The figure shows three views and two pictorial views of one solid part (mm, origin at its lowest corner). Answer the questions. A direction names the side the tool comes from. Give positions to 0.01 mm unless a question says otherwise; leave off trailing zeros. Order: outer loops, then holes, each group sorted by start corner. A loop starts at its lowest first (then second) coordinate and runs counter-clockwise, first axis right, second up. Notation, with made-up numbers: (8.5, 0.25) - (40.5, 0.25) arc R15 ccw to (40.5, 5.25) - close; hole circle Ø11 at (-1.75, 50). An arc over 180 degrees is marked (long way). Write item = value, one per line.
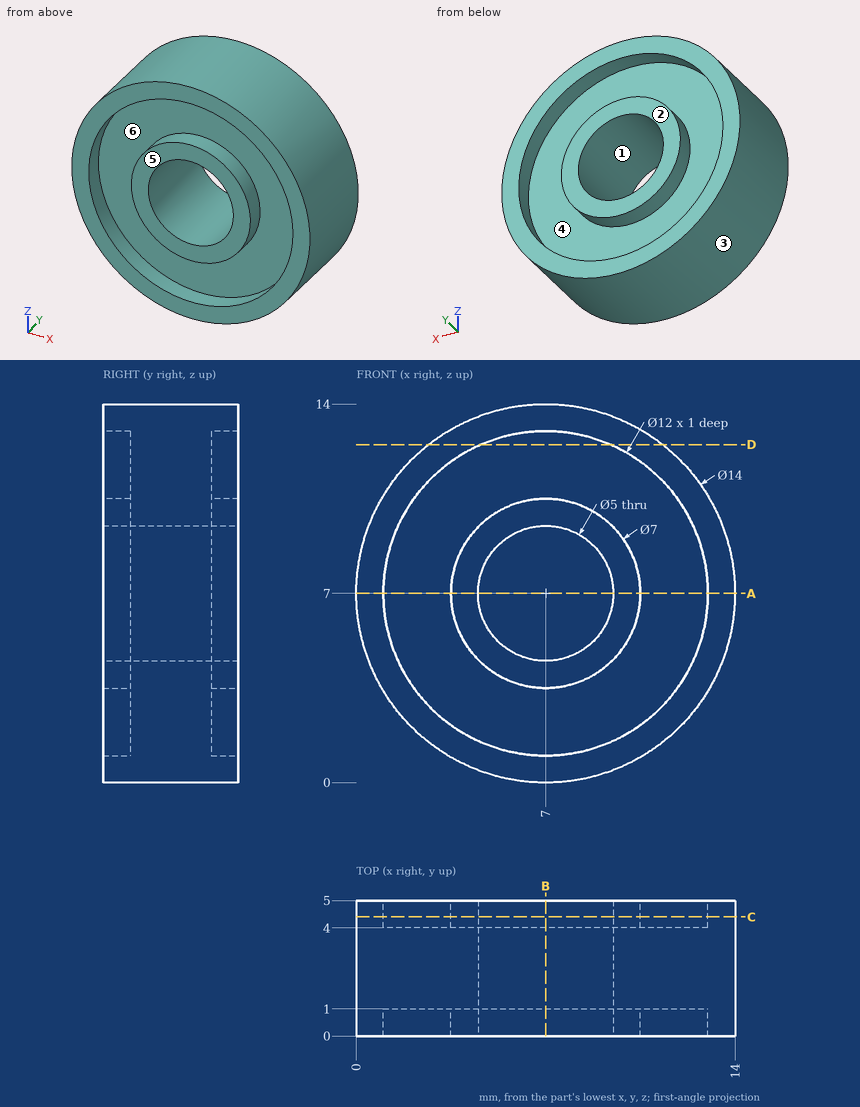
1. Section C-C (y = 4.4) is taken. Determine the outline of the cut face in (x, z).
Recorded:
outline = circle Ø14 at (7, 7); circle Ø7 at (7, 7); hole circle Ø12 at (7, 7); hole circle Ø5 at (7, 7)
2. Straight lines are drawn through the part: L1, parallel to X at y = 4.3, z = 7; L2, parallel to X at y = 4.6, z = 6.5; L3, parallel to X at y = 2.85, z = 7. For each, find the intervals that lie inside material, in ascending order. Write a range as [from, to].
Recorded:
L1 = [0, 1], [3.5, 4.5], [9.5, 10.5], [13, 14]
L2 = [0.02, 1.02], [3.54, 4.55], [9.45, 10.46], [12.98, 13.98]
L3 = [0, 4.5], [9.5, 14]
3. Section D-D (z = 12.5) is taken. Determine the outline of the cut face in (x, y).
Recorded:
outline = (2.67, 0) - (4.6, 0) - (4.6, 1) - (9.4, 1) - (9.4, 0) - (11.33, 0) - (11.33, 5) - (9.4, 5) - (9.4, 4) - (4.6, 4) - (4.6, 5) - (2.67, 5) - close
4. For the marked faces 4, 5 and 6, determine the directions among +Z, -Z, +X, -X, +Y, -Y from which every point of the face is accessible in a straight line to the end or side of a thin tool.
Recorded:
face_4 = +Y
face_5 = +Z, -Z, +X, -X, -Y
face_6 = -Y
5. Flat-ended cylindrical pins translate along their axes: pin 1 (1 mm diameter, centred on y = 3.5, z = 12, fed in from -X); pin 2 (3 mm diameter, centred on x = 4, y = 3, fed in from +Z). Find the tip coordinate at first contact, or state that the pin passes through.
Recorded:
pin_1 = 1.64
pin_2 = 13.84
6. Section B-B (x = 7) is taken. Determine the outline of the cut face in (y, z).
Recorded:
outline = (0, 0) - (5, 0) - (5, 1) - (4, 1) - (4, 3.5) - (5, 3.5) - (5, 4.5) - (0, 4.5) - (0, 3.5) - (1, 3.5) - (1, 1) - (0, 1) - close; (0, 9.5) - (5, 9.5) - (5, 10.5) - (4, 10.5) - (4, 13) - (5, 13) - (5, 14) - (0, 14) - (0, 13) - (1, 13) - (1, 10.5) - (0, 10.5) - close
7. Determine the mould class of the marked faces 1, 2 and 3 for opening direction Z: +Z half, -Z half, draft (parallel to the pull), parting line (faces both ways), or undercut.
Recorded:
face_1 = undercut
face_2 = draft
face_3 = parting line
8. Section A-A (z = 7) is taken. Determine the outline of the cut face in (x, y), and give its area (3 significant figures).
Recorded:
outline = (0, 0) - (1, 0) - (1, 1) - (3.5, 1) - (3.5, 0) - (4.5, 0) - (4.5, 5) - (3.5, 5) - (3.5, 4) - (1, 4) - (1, 5) - (0, 5) - close; (9.5, 0) - (10.5, 0) - (10.5, 1) - (13, 1) - (13, 0) - (14, 0) - (14, 5) - (13, 5) - (13, 4) - (10.5, 4) - (10.5, 5) - (9.5, 5) - close
area = 35.0 mm^2
